Work out the finished part from the listing and answer in its coordinate system (mm). Face numbers are marked on the shaded views. A direction names the side the tool comes from. Round coordinates to 2 decimals unless told otherwise and drop trailing zeros. Loops run counter-clockwise (first coordinate to the right, second up) from the corner with the lowest first, then second, coordinate; pieces in that order, holes last. Notation, with made-up numbers: (-36.5, 23) -> (19.5, 23) arc R11 cw to (19.5, 41) -> close; hole circle Ø4 at (64.5, 83.25). An arc over 180 degrees is marked (long way). Use one line per item in the form item = value.
```python
from build123d import *

# Parameters (mm, degrees)
F0_W        = 155
F0_H        = 151
F1_DEPTH    = 37
F2_T1_DEPTH = 362.8505669038
F3_T        = -2.54
F4_W        = 125.55387271
F4_H        = 111.9176980871
F5_DEPTH    = 25.4
F6_R        = 3.175
F7_DEPTH    = 155.001
F9_DEPTH    = 152.46


# Not quite as in the source:
# - a fillet or chamfer that OpenCascade refuses, or shapes differently, is made with other operations: its cross-section is extruded or revolved along the edge and cut away or added


with BuildPart() as f1:
    # F0 (on Front) → F1 (new body)
    with BuildSketch(Plane.XZ):
        Rectangle(F0_W, F0_H)
    extrude(amount=F1_DEPTH)

    # F2: chamfer of 40 x 8 on 1 edges, made by hand

    # F2_s2 → F2_t1 (cut)
    with BuildSketch(Plane.YZ.offset(-181.4252834519)):
        Polygon((-40, -75.5), (0, -67.5), (0, -75.5), align=None)
    extrude(amount=F2_T1_DEPTH, mode=Mode.SUBTRACT)

    # F3
    f3_openings = [f1.faces().sort_by_distance(p)[0] for p in [
        (0, -37, 0.3),
    ]]
    offset(amount=F3_T, openings=f3_openings)

    # F4 (on face) → F5 (cut)
    with BuildSketch(Plane.XZ.offset(2.54)):
        with Locations((-0.276936355, 9.5411509565)):
            Rectangle(F4_W, F4_H)
    extrude(amount=-F5_DEPTH, mode=Mode.SUBTRACT)

    # F6 (on face) → F7 (cut, through all)
    with BuildSketch(Plane(origin=(-77.5, 0, 0), x_dir=(0, -1, 0), z_dir=(-1, 0, 0))):
        with Locations((21.3561020792, 0)):
            Circle(F6_R)
        with Locations((21.3561020792, 35)):
            Circle(F6_R)
        with Locations((21.3561020792, -30)):
            Circle(F6_R)
    extrude(amount=-F7_DEPTH, mode=Mode.SUBTRACT)

    # F8 (on face) → F9 (join, through all)
    with BuildSketch(Plane(origin=(74.96, 0, 0), x_dir=(0, -1, 0), z_dir=(-1, 0, 0))):
        Polygon((0, -29.1507557497), (37, -47.1048012634), (37, -44.281557044), (0, -26.3275115302), align=None)
        Polygon((0, -2.9595115302), (37, -20.913557044), (37, -18.0903128246), (0, -0.1362673108), align=None)
        Polygon((0, 23.2317326892), (37, 5.2776871754), (37, 8.1009313948), (0, 26.0549769086), align=None)
        Polygon((0, 49.4229769086), (37, 31.4689313948), (37, 34.2921756143), (0, 52.246221128), align=None)
    extrude(amount=F9_DEPTH)


solid = f1.part
```
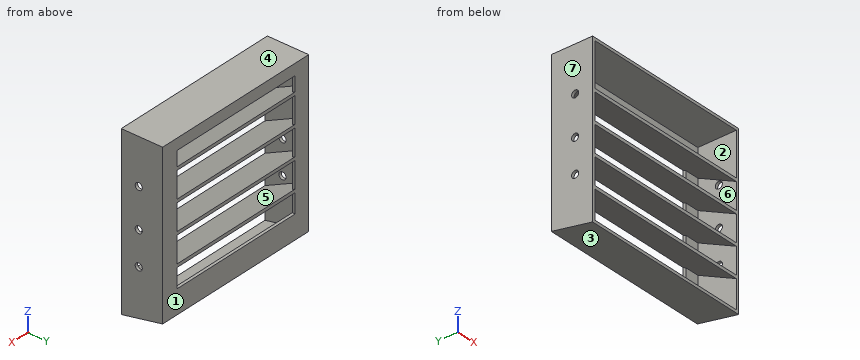
(1) Find section A-A, the plane x = -47.5. Write down the section's boundary in (y, z).
Completed:
outline = (-37, -74.9) -> (0, -67.5) -> (0, -46.42) -> (-2.54, -46.42) -> (-2.54, -65.42) -> (-37, -72.31) -> close; (-37, -47.1) -> (0, -29.15) -> (0, -26.33) -> (-37, -44.28) -> close; (-37, -20.91) -> (0, -2.96) -> (0, -0.14) -> (-37, -18.09) -> close; (-37, 5.28) -> (0, 23.23) -> (0, 26.05) -> (-37, 8.1) -> close; (-37, 31.47) -> (0, 49.42) -> (0, 52.25) -> (-37, 34.29) -> close; (-37, 72.96) -> (-2.54, 72.96) -> (-2.54, 65.5) -> (0, 65.5) -> (0, 75.5) -> (-37, 75.5) -> close
(2) For a pull along Z with two mould halves and no side action, classify the marked faces 1, 2, 3 and 4 as +Z half, -Z half, draft (parallel to the pull), parting line (faces both ways), or undercut.
Completed:
face_1 = draft
face_2 = undercut
face_3 = -Z half
face_4 = +Z half
(3) Consider L1, parallel to X at y = -7, z = 39; L2, parallel to Z at x = 20, y = -29; L3, parallel to Z at x = 68, y = -6.5. Determine where each line is inside the solid, lowest interval first.
Completed:
L1 = -77.5 to -74.96, 74.96 to 77.5
L2 = -73.3 to -70.71, -43.22 to -40.4, -17.03 to -14.21, 9.16 to 11.98, 35.35 to 38.17, 72.96 to 75.5
L3 = -68.8 to -66.21, -32.3 to -29.48, -6.11 to -3.29, 20.08 to 22.9, 46.27 to 49.09, 72.96 to 75.5
(4) Given P1, Ø8.5, axis at y = -21.36, z = 35, coming from the -X side; P2, Ø4, axis at x = 30, y = -20.5, coming from the -Z side; P3, Ø8, axis at x = -29, y = -24, coming from the -Z side; P4, Ø12, axis at x = -27, z = -27.5, coming from the -Y side, each flat-ended and moving along its own axis, determine where each tip first touches the part or whether it passes through.
Completed:
P1 = -77.5
P2 = -72
P3 = -73.1
P4 = -14.78
(5) Find section B-B, the plane z = 56. Write down the section's boundary in (x, y), then the cut area to 3 significant figures.
Completed:
outline = (-77.5, -37) -> (-74.96, -37) -> (-74.96, -2.54) -> (-63.05, -2.54) -> (-63.05, 0) -> (-77.5, 0) -> close; (62.5, -2.54) -> (74.96, -2.54) -> (74.96, -37) -> (77.5, -37) -> (77.5, 0) -> (62.5, 0) -> close
area = 250 mm2
(6) Find section D-D, the plane y = -14. Write down the section's boundary in (x, z).
Completed:
outline = (-77.5, -70.3) -> (77.5, -70.3) -> (77.5, 75.5) -> (-77.5, 75.5) -> close; hole (-74.96, -67.71) -> (74.96, -67.71) -> (74.96, -35.94) -> (-74.96, -35.94) -> close; hole (-74.96, -33.12) -> (74.96, -33.12) -> (74.96, -9.75) -> (-74.96, -9.75) -> close; hole (-74.96, -6.93) -> (74.96, -6.93) -> (74.96, 16.44) -> (-74.96, 16.44) -> close; hole (-74.96, 19.26) -> (74.96, 19.26) -> (74.96, 42.63) -> (-74.96, 42.63) -> close; hole (-74.96, 45.45) -> (74.96, 45.45) -> (74.96, 72.96) -> (-74.96, 72.96) -> close
(7) For the marked faces 5, 6 and 7, determine the directions among +Z, -Z, +X, -X, +Y, -Y from which every point of the face is accessible in a straight line to the end or side of a thin tool.
Completed:
face_5 = -Y
face_6 = none
face_7 = +Z, -Z, -X, +Y, -Y
(8) Find section C-C, the plane y = -34. Write down the section's boundary in (x, z), then the cut area to 3 significant figures.
Completed:
outline = (-77.5, -74.3) -> (77.5, -74.3) -> (77.5, 75.5) -> (-77.5, 75.5) -> close; hole (-74.96, -71.71) -> (74.96, -71.71) -> (74.96, -45.65) -> (-74.96, -45.65) -> close; hole (-74.96, -42.83) -> (74.96, -42.83) -> (74.96, -19.46) -> (-74.96, -19.46) -> close; hole (-74.96, -16.63) -> (74.96, -16.63) -> (74.96, 6.73) -> (-74.96, 6.73) -> close; hole (-74.96, 9.56) -> (74.96, 9.56) -> (74.96, 32.92) -> (-74.96, 32.92) -> close; hole (-74.96, 35.75) -> (74.96, 35.75) -> (74.96, 72.96) -> (-74.96, 72.96) -> close
area = 3,220 mm2
